Input: part model. Units: mm. Frame: model coordinates. A direction names the side the tool comes from. Give positions to 0.01 mm unless a question says otherwise; leave off trailing zeros. Loops run counter-clockwise (first coordinate to the right, second up) from the corner with the lowest first, then second, coordinate; pieces in that order, holes last.
from build123d import *

# Parameters (mm, degrees)
F0_W      = 53.943
F0_H      = 41.85567
F1_DEPTH  = 5
F2_R      = 18.466
F3_DEPTH  = 5
F4_R      = 14.344
F5_DEPTH  = 5
F6_R      = 9.61
F7_DEPTH  = 5
F8_R      = 5.8635
F9_DEPTH  = 5
F10_R     = 3.3955
F11_DEPTH = 25.001


with BuildPart() as f1:
    # F0 (on Front) → F1 (new body)
    with BuildSketch(Plane.XZ):
        Rectangle(F0_W, F0_H)
    extrude(amount=F1_DEPTH)

    # F2 (on face) → F3 (join)
    with BuildSketch(Plane.XZ.offset(5)):
        Circle(F2_R)
    extrude(amount=F3_DEPTH)

    # F4 (on face) → F5 (join)
    with BuildSketch(Plane.XZ.offset(10)):
        Circle(F4_R)
    extrude(amount=F5_DEPTH)

    # F6 (on face) → F7 (join)
    with BuildSketch(Plane.XZ.offset(15)):
        Circle(F6_R)
    extrude(amount=F7_DEPTH)

    # F8 (on face) → F9 (join)
    with BuildSketch(Plane.XZ.offset(20)):
        Circle(F8_R)
    extrude(amount=F9_DEPTH)

    # F10 (on face) → F11 (cut, through all)
    with BuildSketch(Plane.XZ.offset(25)):
        Circle(F10_R)
    extrude(amount=-F11_DEPTH, mode=Mode.SUBTRACT)


solid = f1.part
(1) Cut plane A-A (z = 0). Return the cut outline in (x, y).
Values follow:
outline: (-26.97, -5) - (-18.47, -5) - (-18.47, -10) - (-14.34, -10) - (-14.34, -15) - (-9.61, -15) - (-9.61, -20) - (-5.86, -20) - (-5.86, -25) - (-3.4, -25) - (-3.4, 0) - (-26.97, 0) - close; (3.4, -25) - (5.86, -25) - (5.86, -20) - (9.61, -20) - (9.61, -15) - (14.34, -15) - (14.34, -10) - (18.47, -10) - (18.47, -5) - (26.97, -5) - (26.97, 0) - (3.4, 0) - close
(2) Cut plane D-D (x = -20). Return the cut outline in (y, z).
Values follow:
outline: (-5, -20.93) - (0, -20.93) - (0, 20.93) - (-5, 20.93) - close
(3) Ray query, probe 1 along Z at (x, y) = (0, -18.75); probe 2 along Z at (x, y) = (0, -9.75); probe 3 along Y at (x, z) = (23, 1). Return the intervals inside material, ascending.
Values follow:
probe 1: z = -9.61 to -3.4, 3.4 to 9.61
probe 2: z = -18.47 to -3.4, 3.4 to 18.47
probe 3: y = -5 to 0
(4) Cut plane C-C (y = -22.25). Return the cut outline in (x, z).
Values follow:
outline: circle Ø11.73 at (0, 0); hole circle Ø6.79 at (0, 0)
(5) Reachability of faces 1 (the flat face through (-4.4, -20, -4.1)), 2 (the flat face through (0, -2, -20.928)) from +Z, -Z, +X, -X, +Y, -Y: full face, straight path, thin tool, end or side. Return the list, or none.
Values follow:
face 1: -Y
face 2: -Z, +X, -X, +Y, -Y
(6) Pin query (flat end, axial travel): pin 1 Ø1.5 at (x, y) = (0.5, -14.5) entering from -Z; pin 2 Ø2 at (x, z) = (-10.5, 2.5) entering from -Y; pin 3 Ø5 at (x, y) = (-10, -8.5) entering from +Z; pin 4 Ø4 at (x, z) = (0, 0) entering from +Y. Return the tip coordinate at first contact, or that it passes through.
Values follow:
pin 1: stops at z = -14.34
pin 2: stops at y = -15
pin 3: stops at z = 16.87
pin 4: passes through
(7) Cut plane B-B (x = 0). Return the cut outline in (y, z), and give its area (3 significant figures).
Values follow:
outline: (-25, -5.86) - (-20, -5.86) - (-20, -9.61) - (-15, -9.61) - (-15, -14.34) - (-10, -14.34) - (-10, -18.47) - (-5, -18.47) - (-5, -20.93) - (0, -20.93) - (0, -3.4) - (-25, -3.4) - close; (-25, 3.4) - (0, 3.4) - (0, 20.93) - (-5, 20.93) - (-5, 18.47) - (-10, 18.47) - (-10, 14.34) - (-15, 14.34) - (-15, 9.61) - (-20, 9.61) - (-20, 5.86) - (-25, 5.86) - close
area: 522 mm2
